Autodesk Inventor part; units mm, degrees
ref_plane "YZ Plane" through (0, 0, 0) normal (1, 0, 0) x (0, 1, 0)
ref_plane "XZ Plane" through (0, 0, 0) normal (0, 1, 0) x (-1, 0, 0)
ref_plane "XY Plane" through (0, 0, 0) normal (0, 0, 1) x (1, 0, 0)
sketch "Sketch1" plane through (0, 0, 0) normal (0, 1, 0) x (-1, 0, 0)
  line L0 (-4.0561, -5.7426) -> (-4.0561, 5.2574)
  line L1 (-3.0561, 6.2574) -> (2.9439, 6.2574)
  line L2 (3.9439, 5.2574) -> (3.9439, -5.7426)
  line L3 (3.9439, -5.7426) -> (1.9439, -5.7426)
  line L4 (1.9439, -5.7426) -> (1.9439, 2.2574)
  line L5 (0.9439, 3.2574) -> (-1.0561, 3.2574)
  line L6 (-2.0561, 2.2574) -> (-2.0561, -5.7426)
  line L7 (-2.0561, -5.7426) -> (-4.0561, -5.7426)
  arc A0 (-1.0561, 3.2574) -> (-2.0561, 2.2574) centre (-1.0561, 2.2574) ccw
  arc A1 (1.9439, 2.2574) -> (0.9439, 3.2574) centre (0.9439, 2.2574) ccw
  arc A2 (-3.0561, 6.2574) -> (-4.0561, 5.2574) centre (-3.0561, 5.2574) ccw
  arc A3 (3.9439, 5.2574) -> (2.9439, 6.2574) centre (2.9439, 5.2574) ccw
  point P0 (0, 0)
  point P1 (-4.0561, 6.2574)
  point P2 (3.9439, 6.2574)
  point P3 (1.9439, 3.2574)
  point P4 (-2.0561, 3.2574)
  dimension "d0" = 12
  dimension "d1" = 2
  dimension "d2" = 2
  dimension "d3" = 8
  dimension "d4" = 3
  dimension "d20" = 1
extrude "Extrusion1" add sketch "Sketch1" along normal blind 10
sketch "Sketch6" plane through (-1.9439, 0, 2.2574) normal (1, 0, 0) x (0, 0, -1)
  circle A0 centre (2, 2) radius 1
  circle A1 centre (6, 2) radius 1
  line L0 (8, 0) -> (8, 10)
  line L1 (0, 10) -> (8, 10)
  line L2 (8, 0) -> (0, 0)
  point P0 (2.2574, 0)
  dimension "d44" = 2
  dimension "d45" = 2
  dimension "d46" = 2
  dimension "d47" = 6
  dimension "d52" = 2
  dimension "d53" = 2
extrude "Extrusion6" cut sketch "Sketch6" against normal up to next
sketch "Sketch7" plane through (4.0561, 0, 5.2574) normal (1, 0, 0) x (0, 0, -1)
  line L0 (4, 10) -> (4, 9)
  line L1 (4, 9) -> (7, 9)
  line L2 (7, 9) -> (7, 10)
  line L3 (0, 10) -> (11, 10)
  line L4 (11, 0) -> (11, 10)
  line L5 (0, 0) -> (0, 10)
  line L6 (4, 10) -> (7, 10)
  point P0 (5.2574, 0)
  dimension "d54" = 4
  dimension "d55" = 4
  dimension "d57" = 1
extrude "Extrusion7" cut sketch "Sketch7" against normal up to next
sketch "Sketch8" plane through (4.0561, 0, 5.2574) normal (1, 0, 0) x (0, 0, -1)
  line L0 (0, 0) -> (0, 10)
  line L1 (0, 5) -> (4, 5)
  line L2 (4, 5) -> (4, 6)
  line L3 (4, 6) -> (7, 6)
  line L4 (7, 6) -> (7, 5)
  line L5 (7, 5) -> (11, 5)
  line L6 (11, 0) -> (11, 10)
  line L7 (11, 5) -> (11, 0)
  line L8 (11, 0) -> (0, 0)
  line L9 (0, 0) -> (0, 5)
  point P0 (5.2574, 0)
  dimension "d60" = 5
  dimension "d61" = 1
  dimension "d62" = 4
  dimension "d63" = 4
extrude "Extrusion8" cut sketch "Sketch8" against normal up to surface (2 mm away)
properties part number "crochet"
The model under review builds one solid part; all positions refer to its coordinate system, in mm. A direction names the side the tool comes from. Give positions to 0.01 mm unless a question says otherwise; leave off trailing zeros. Order: outer loops, then holes, each group sorted by start corner. A loop starts at its lowest first (then second) coordinate and runs counter-clockwise, first axis right, second up. Notation, with made-up numbers: M 59,86 L 70,86 A21 ccw 70,111 Z; hole C 63,-33.75 d8. An arc over 180 degrees is marked long. Answer in a Markdown table with one row per item. Add a question column.
1. Add section D-D on y = 7.5. State the section outline as (x, z) points.
2. For pin 1 Ø1.6 at (x, z) = (3, -0.5) entering from -Y; pin 2 Ø1.6 at (y, z) = (2, -3.74) entering from +X; pin 3 Ø2 at (x, z) = (3, -3.5) entering from -Y, all flat-tipped, find the tip position at first contact; note any pin that passes through.
3. Add section C-C on z = -4.5. State the section outline as (x, y) points.
4. To check wall thickness, follow line 1 along X through (y, z) = (6.25, -2.5); line 2 along Z through (x, y) = (2.75, 5.5); line 3 along X through (y, z) = (2.5, -1.75). State the ranges of each line that lie inside material, in increasing order.
5. Add section B-B on z = -1. State the section outline as (x, y) points, plus the area to 3 significant figures.
6. Machinability: for faces 1 (the flat face through (3.1, 9.5, 1.257)), 2 (the flat face through (3, 5, 3)), 3 (the flat face through (3.1, 5.5, -1.743)), 4 (the cylindrical face through (1.77, 4.93, 2.96)), which of the approach directions +Z, -Z, +X, -X, +Y, -Y give a long, thin tool a straight path to every point of the face, cutting with its end or side? Answer none if there is none.
7. Add section A-A on y = 2. State the section outline as (x, z) points, plus the area to 3 significant figures.
8. Mouldability with a two-part tool opening along X and no side actions: class faces 5 (the flat face through (2.056, 7, -2)), 6 (the cylindrical face through (-1.643, 4.93, 2.972)), 7 (the flat face through (4.056, 7, 0)), 8 (the flat face through (0, 5, 6.257)) as released by +X, released by -X, zero draft, split by the parting line, or undercut.
The answers:
| question | item | result |
|---|---|---|
| 1 | outline | M -3.94,-5.74 L -1.94,-5.74 L -1.94,2.26 A1 cw -0.94,3.26 L 1.06,3.26 A1 cw 2.06,2.26 L 2.06,-5.74 L 4.06,-5.74 L 4.06,5.26 A1 ccw 3.06,6.26 L -2.94,6.26 A1 ccw -3.94,5.26 Z |
| 2 | pin 1 | y = 6 |
| 2 | pin 2 | through |
| 2 | pin 3 | y = 5 |
| 3 | outline | M -3.94,0 L -1.94,0 L -1.94,1.35 L -3.94,1.35 Z; M -3.94,2.65 L -1.94,2.65 L -1.94,10 L -3.94,10 Z; M 2.06,5 L 4.06,5 L 4.06,10 L 2.06,10 Z |
| 4 | line 1 | -3.94 to -1.94, 2.06 to 4.06 |
| 4 | line 2 | -5.74 to -1.74, 1.26 to 6.26 |
| 4 | line 3 | -3.94 to -1.94 |
| 5 | outline | M -3.94,0 L -1.94,0 L -1.94,10 L -3.94,10 Z; M 2.06,6 L 4.06,6 L 4.06,9 L 2.06,9 Z |
| 5 | area | 26.0 mm2 |
| 6 | face 1 | +X, +Y |
| 6 | face 2 | -Z, +X, -Y |
| 6 | face 3 | +X, -Y |
| 6 | face 4 | -Z, +Y, -Y |
| 7 | outline | M -3.94,-5.74 L -1.94,-5.74 L -1.94,-4.74 L -3.94,-4.74 Z; M -3.94,-2.74 L -1.94,-2.74 L -1.94,-0.74 L -3.94,-0.74 Z; M -3.94,1.26 L -1.94,1.26 L -1.94,2.26 A1 cw -0.94,3.26 L 1.06,3.26 A1 cw 2.06,2.26 L 2.06,5.26 L 4.06,5.26 A1 ccw 3.06,6.26 L -2.94,6.26 A1 ccw -3.94,5.26 Z |
| 7 | area | 30.0 mm2 |
| 8 | face 5 | undercut |
| 8 | face 6 | undercut |
| 8 | face 7 | released by +X |
| 8 | face 8 | zero draft |
